Geometry check sheet. Reference: the model listing, model coordinates, mm. A direction names the side the tool comes from. Coordinates: 2 decimals unless noted, no trailing zeros. Order: outer loops, then holes, each group sorted by start corner. A loop starts at its lowest first (then second) coordinate and runs counter-clockwise, first axis right, second up. Notation, with made-up numbers: (31.5, 78.5) - (53.5, 78.5) arc R21 cw to (53.5, 92.5) - close; hole circle Ø4 at (54, -30.75). An arc over 180 degrees is marked (long way). Put each result on its own line as item: value.
from build123d import *

# Parameters (mm, degrees)
CROQUIS1_R              = 17.5
CROQUIS1_R_2            = 1.52
SALIENTE_EXTRUIR1_DEPTH = 3
CROQUIS2_R              = 10
CROQUIS2_R_2            = 1.5
SALIENTE_EXTRUIR2_DEPTH = 10


with BuildPart() as part:
    # Croquis1 → Saliente-Extruir1 (new body)
    with BuildSketch(Plane(origin=(0, 0, 0), x_dir=(1, 0, 0), z_dir=(0, 1, 0))):
        with Locations(Location((0, 0, 0), (0, 0, 270))):
            Circle(CROQUIS1_R)
        with Locations(Location((12.5, 0, 0), (0, 0, 270))):
            Circle(CROQUIS1_R_2, mode=Mode.SUBTRACT)
        with Locations(Location((6.25, -10.825317547, 0), (0, 0, 270))):
            Circle(CROQUIS1_R_2, mode=Mode.SUBTRACT)
        with Locations(Location((-6.25, -10.825317547, 0), (0, 0, 270))):
            Circle(CROQUIS1_R_2, mode=Mode.SUBTRACT)
        with Locations(Location((-12.5, 0, 0), (0, 0, 270))):
            Circle(CROQUIS1_R_2, mode=Mode.SUBTRACT)
        with Locations(Location((-6.25, 10.825317547, 0), (0, 0, 270))):
            Circle(CROQUIS1_R_2, mode=Mode.SUBTRACT)
        with Locations(Location((6.25, 10.825317547, 0), (0, 0, 270))):
            Circle(CROQUIS1_R_2, mode=Mode.SUBTRACT)
    extrude(amount=SALIENTE_EXTRUIR1_DEPTH)

    # Croquis2 → Saliente-Extruir2 (add)
    with BuildSketch(Plane(origin=(0, 3, 0), x_dir=(1, 0, 0), z_dir=(0, 1, 0))):
        with Locations(Location((0, 0, 0), (0, 0, 270))):
            Circle(CROQUIS2_R)
        with Locations(Location((7.5, 0, 0), (0, 0, 270))):
            Circle(CROQUIS2_R_2, mode=Mode.SUBTRACT)
        with Locations(Location((3.75, -6.495190528, 0), (0, 0, 270))):
            Circle(CROQUIS2_R_2, mode=Mode.SUBTRACT)
        with Locations(Location((-3.75, -6.495190528, 0), (0, 0, 270))):
            Circle(CROQUIS2_R_2, mode=Mode.SUBTRACT)
        with Locations(Location((-7.5, 0, 0), (0, 0, 270))):
            Circle(CROQUIS2_R_2, mode=Mode.SUBTRACT)
        with Locations(Location((-3.75, 6.495190528, 0), (0, 0, 270))):
            Circle(CROQUIS2_R_2, mode=Mode.SUBTRACT)
        with Locations(Location((3.75, 6.495190528, 0), (0, 0, 270))):
            Circle(CROQUIS2_R_2, mode=Mode.SUBTRACT)
    extrude(amount=SALIENTE_EXTRUIR2_DEPTH)


solid = part.part
Q1. Section check D-D on x = 12.5. Record the boundary of the cut face in (y, z), then the cut area to 3 significant figures.
Answer block:
outline: (0, -12.25) - (3, -12.25) - (3, -1.52) - (0, -1.52) - close; (0, 1.52) - (3, 1.52) - (3, 12.25) - (0, 12.25) - close
area: 64.4 mm^2
Q2. Thickness scan on L1, parallel to X at y = 9.75, z = 0; L2, parallel to X at y = 1, z = 0; L3, parallel to Y at x = -12, z = 4. Record the ranges inside material, lowest first. Write a range as [from, to].
Answer block:
L1: x = [-10, -9], [-6, 6], [9, 10]
L2: x = [-17.5, -14.02], [-10.98, 10.98], [14.02, 17.5]
L3: y = [0, 3]
Q3. Section check A-A on z = 0. Record the boundary of the cut face in (x, y).
Answer block:
outline: (-17.5, 0) - (-14.02, 0) - (-14.02, 3) - (-17.5, 3) - close; (-10.98, 0) - (10.98, 0) - (10.98, 3) - (10, 3) - (10, 13) - (9, 13) - (9, 3) - (6, 3) - (6, 13) - (-6, 13) - (-6, 3) - (-9, 3) - (-9, 13) - (-10, 13) - (-10, 3) - (-10.98, 3) - close; (14.02, 0) - (17.5, 0) - (17.5, 3) - (14.02, 3) - close
Q4. Section check C-C on x = 0. Record the boundary of the cut face in (y, z), then the cut area to 3 significant figures.
Answer block:
outline: (0, -17.5) - (3, -17.5) - (3, -10) - (13, -10) - (13, 10) - (3, 10) - (3, 17.5) - (0, 17.5) - close
area: 305 mm^2
Q5. Access from +Z, -Z, +X, -X, +Y, -Y to the whole of each face (thin tool, end or side, straight path). Record for faces 1 (the cylindrical face through (-10.993, 1.479, -0.198)), 2 (the flat face through (4, 3, -7)).
Answer block:
face 1: +Y, -Y
face 2: +Y
Q6. Draft check along X on faces 3 (the cylindrical face through (-7.175, 1.479, -12.032)), 4 (the flat face through (-8, 3, 8)), 5 (the cylindrical face through (-10.648, 1.479, -13.887)). Enter one of: pulls with the +X half, pulls with the -X half, needs draft (parallel to the pull), parting line crosses it, or undercut.
Answer block:
face 3: undercut
face 4: needs draft
face 5: parting line crosses it
Q7. Depth check by flat-ended pin: pin 1 Ø2.5 at (x, z) = (-7.5, -0.5) entering from +Y; pin 2 Ø2 at (x, y) = (-3.5, 9) entering from +Z; pin 3 Ø1.5 at (x, y) = (-3.5, 10.5) entering from +Z; pin 4 Ø5 at (x, y) = (9.5, 11.5) entering from +Z. Enter the tip coordinate at first touch or a pass-through.
Answer block:
pin 1: stops at y = 13
pin 2: stops at z = 9.68
pin 3: stops at z = 9.61
pin 4: stops at z = 7.14
Q8. Section check B-B on y = 1.75. Record the boundary of the cut face in (x, z), then the cut area to 3 significant figures.
Answer block:
outline: circle Ø35 at (0, 0); hole circle Ø3.04 at (-12.5, 0); hole circle Ø3.04 at (-6.25, -10.83); hole circle Ø3.04 at (-6.25, 10.83); hole circle Ø3.04 at (6.25, -10.83); hole circle Ø3.04 at (6.25, 10.83); hole circle Ø3.04 at (12.5, 0)
area: 919 mm^2
